```python
from build123d import *

# Parameters (mm, degrees)
SURFACE_EXTRUDE1_1_DEPTH = 450
THICKEN15_T2             = 1.2
SKETCH2_R                = 25
CUT_EXTRUDE1_DEPTH       = 10
SKETCH3_R                = 2.5
CUT_EXTRUDE2_DEPTH       = 10


with BuildPart() as body_1:
    # Surface-Extrude1: a surface, the sketch's curves swept straight by 450 mm
    with BuildLine(Plane(origin=(0, 0, 0), x_dir=(0, 0, -1), z_dir=(1, 0, 0)), mode=Mode.PRIVATE) as surface_extrude1_1_path:
        Line((0, 0), (0, 210))
    surface_extrude1_1 = Shell.extrude(surface_extrude1_1_path.wire(), (1 * SURFACE_EXTRUDE1_1_DEPTH, 0 * SURFACE_EXTRUDE1_1_DEPTH, 0 * SURFACE_EXTRUDE1_1_DEPTH))
    add(Solid.thicken(surface_extrude1_1, -THICKEN15_T2))

    # Sketch2 → Cut-Extrude1 (cut)
    with BuildSketch(Plane.XY):
        with Locations((53, 153)):
            Circle(SKETCH2_R)
    extrude(amount=-CUT_EXTRUDE1_DEPTH, mode=Mode.SUBTRACT)

    # Sketch3 → Cut-Extrude2 (cut)
    with BuildSketch(Plane.XY):
        with Locations((10, 60)):
            Circle(SKETCH3_R)
        with Locations((10, 105)):
            Circle(SKETCH3_R)
        with Locations((10, 150)):
            Circle(SKETCH3_R)
        with Locations(Location((440, 60, 0), (0, 0, 180))):
            Circle(SKETCH3_R)
        with Locations(Location((440, 105, 0), (0, 0, 180))):
            Circle(SKETCH3_R)
        with Locations(Location((440, 150, 0), (0, 0, 180))):
            Circle(SKETCH3_R)
        with Locations((60, 200)):
            Circle(SKETCH3_R)
        with Locations((150, 200)):
            Circle(SKETCH3_R)
        with Locations(Location((300, 200, 0), (0, 0, 180))):
            Circle(SKETCH3_R)
        with Locations(Location((390, 200, 0), (0, 0, 180))):
            Circle(SKETCH3_R)
        with Locations((390, 10)):
            Circle(SKETCH3_R)
        with Locations((300, 10)):
            Circle(SKETCH3_R)
        with Locations(Location((150, 10, 0), (0, 0, 180))):
            Circle(SKETCH3_R)
        with Locations(Location((60, 10, 0), (0, 0, 180))):
            Circle(SKETCH3_R)
    extrude(amount=-CUT_EXTRUDE2_DEPTH, mode=Mode.SUBTRACT)


solid = body_1.part
```
The listing builds one solid part. Answer for the finished solid, in the listing's coordinates (mm). Give positions to 0.01 mm unless a question says otherwise; leave off trailing zeros. Order: outer loops, then holes, each group sorted by start corner. A loop starts at its lowest first (then second) coordinate and runs counter-clockwise, first axis right, second up.
1) Find section B-B on z = -0.3. Give the number of separate pieces and of enclosed holes in the cut face, then the cut area to 3 significant figures.
Reported:
separate pieces: 1
enclosed holes: 15
area: 92,300 mm2
2) Given P1, Ø8, axis at x = 300, y = 200, coming from the +Z side; P2, Ø4.5, axis at x = 440, y = 105, coming from the -Z side, each flat-ended and moving along its own axis, determine where each tip first touches the part or whether it passes through.
Reported:
P1: stops at z = 0
P2: passes through
3) Determine the mould class of faces 1 (the face through (49.745, 177.787, -0.592)), 2 (the face through (222, 104, 0)) for opening direction X: pulls with the +X half, pulls with the -X half, needs draft (parallel to the pull), parting line crosses it, or undercut.
Reported:
face 1: undercut
face 2: needs draft
4) Find section A-A on x = 53. Write down the section's boundary in (y, z), then the cut area to 3 significant figures.
Reported:
outline: (0, -1.2) - (128, -1.2) - (128, 0) - (0, 0) - close; (178, -1.2) - (210, -1.2) - (210, 0) - (178, 0) - close
area: 192 mm2
5) Consider line 1 along Y through (x, z) = (440, -0.4); line 2 along X through (y, z) = (200, -0.3); line 3 along Y through (x, z) = (60, -0.3). Determine where each line is inside the solid, lowest interval first.
Reported:
line 1: y = 0 to 57.5, 62.5 to 102.5, 107.5 to 147.5, 152.5 to 210
line 2: x = 0 to 57.5, 62.5 to 147.5, 152.5 to 297.5, 302.5 to 387.5, 392.5 to 450
line 3: y = 0 to 7.5, 12.5 to 129, 177 to 197.5, 202.5 to 210
